from build123d import *

# Parameters (mm, degrees)
SKETCH_W        = 70.3
SKETCH_H        = 51
PAD_DEPTH       = 50.65
SKETCH001_W     = 44.3
SKETCH001_H     = 47.65
SKETCH001_W_2   = 10
POCKET_DEPTH    = 51.001
SKETCH002_R     = 2
SKETCH002_W     = 15
SKETCH002_H     = 15
POCKET001_DEPTH = 50.651


with BuildPart() as part:
    # Sketch → Pad (new body)
    with BuildSketch(Plane.XY):
        with Locations((35.15, 25.5)):
            Rectangle(SKETCH_W, SKETCH_H)
    extrude(amount=PAD_DEPTH)

    # Sketch001 → Pocket (cut, through all)
    with BuildSketch(Plane.XZ):
        with Locations((35.15, 23.825)):
            Rectangle(SKETCH001_W, SKETCH001_H)
        with Locations((5, 26.825)):
            Rectangle(SKETCH001_W_2, SKETCH001_H)
        with Locations((65.3, 26.825)):
            Rectangle(SKETCH001_W_2, SKETCH001_H)
    extrude(amount=-POCKET_DEPTH, mode=Mode.SUBTRACT)

    # Sketch002 → Pocket001 (cut, through all)
    with BuildSketch(Plane.XY.offset(50.65)):
        with Locations((20, 41)):
            Circle(SKETCH002_R)
        with Locations((50.3, 41)):
            Circle(SKETCH002_R)
        with Locations((20, 10)):
            Circle(SKETCH002_R)
        with Locations((50.3, 10)):
            Circle(SKETCH002_R)
        with Locations((4, 40.8)):
            Circle(SKETCH002_R)
        with Locations((4, 30.6)):
            Circle(SKETCH002_R)
        with Locations((4, 20.4)):
            Circle(SKETCH002_R)
        with Locations((4, 10.2)):
            Circle(SKETCH002_R)
        with Locations((66.3, 40.8)):
            Circle(SKETCH002_R)
        with Locations((66.3, 30.6)):
            Circle(SKETCH002_R)
        with Locations((66.3, 20.4)):
            Circle(SKETCH002_R)
        with Locations((66.3, 10.2)):
            Circle(SKETCH002_R)
        with Locations((35.15, 43.5)):
            Rectangle(SKETCH002_W, SKETCH002_H)
    extrude(amount=-POCKET001_DEPTH, mode=Mode.SUBTRACT)


solid = part.part
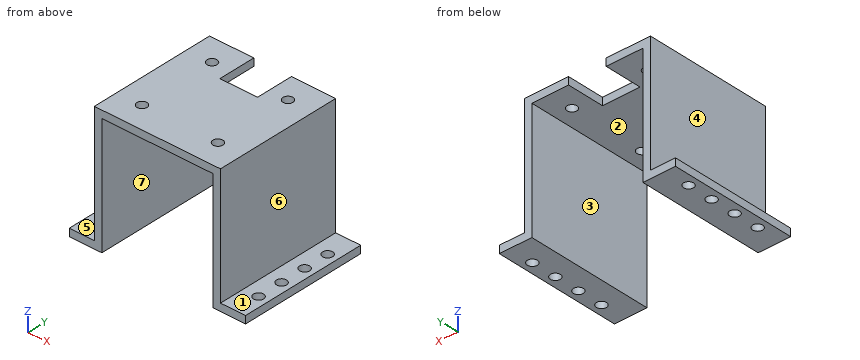
Design review of the part built by this model. Coordinates are the model's own, in mm. Face numbers are marked on the shaded views. A direction names the side the tool comes from. Coordinates: 2 decimals unless noted, no trailing zeros. Order: outer loops, then holes, each group sorted by start corner. A loop starts at its lowest first (then second) coordinate and runs counter-clockwise, first axis right, second up. Notation, with made-up numbers: M 57.25,-16 L 112.25,-16 A26 ccw 112.25,2 Z; hole C -4.75,33 d2. An arc over 180 degrees is marked long. Use a Markdown table: item, result.
(1) Add section C-C (x = 4). Give the boundary of the cut face in (y, z).
Worked answers:
| item | result |
|---|---|
| outline | M 0,0 L 8.2,0 L 8.2,3 L 0,3 Z; M 12.2,0 L 18.4,0 L 18.4,3 L 12.2,3 Z; M 22.4,0 L 28.6,0 L 28.6,3 L 22.4,3 Z; M 32.6,0 L 38.8,0 L 38.8,3 L 32.6,3 Z; M 42.8,0 L 51,0 L 51,3 L 42.8,3 Z |
(2) Draft analysis for pull direction X (two halves, no side actions). For the marked faces 1, 2, 3 and 4, state which applies: released by +X, released by -X, zero draft, split by the parting line, or undercut.
Worked answers:
| item | result |
|---|---|
| face 1 | zero draft |
| face 2 | undercut |
| face 3 | undercut |
| face 4 | released by -X |
(3) Add section B-B (z = 22.5). Give the boundary of the cut face in (x, y), then the cut area to 3 significant figures.
Worked answers:
| item | result |
|---|---|
| outline | M 10,0 L 13,0 L 13,51 L 10,51 Z; M 57.3,0 L 60.3,0 L 60.3,51 L 57.3,51 Z |
| area | 306 mm2 |
(4) Add section D-D (y = 37.5). Give the boundary of the cut face in (x, z).
Worked answers:
| item | result |
|---|---|
| outline | M 0,0 L 13,0 L 13,47.65 L 27.65,47.65 L 27.65,50.65 L 10,50.65 L 10,3 L 0,3 Z; M 42.65,47.65 L 57.3,47.65 L 57.3,0 L 70.3,0 L 70.3,3 L 60.3,3 L 60.3,50.65 L 42.65,50.65 Z |
(5) For the marked faces 5, 6 and 7, list the 3-axis set-ups (+Z, -Z, +X, -X, +Y, -Y) from which the entire face can be reached by the end or side of a thin tool; tool diameter is ignored.
Worked answers:
| item | result |
|---|---|
| face 5 | +Z, -X, +Y, -Y |
| face 6 | +Z, +X, +Y, -Y |
| face 7 | -Z, +Y, -Y |
(6) Add section A-A (y = 30.6). Give the boundary of the cut face in (x, z).
Worked answers:
| item | result |
|---|---|
| outline | M 0,0 L 2,0 L 2,3 L 0,3 Z; M 6,0 L 13,0 L 13,47.65 L 57.3,47.65 L 57.3,0 L 64.3,0 L 64.3,3 L 60.3,3 L 60.3,50.65 L 10,50.65 L 10,3 L 6,3 Z; M 68.3,0 L 70.3,0 L 70.3,3 L 68.3,3 Z |
(7) For P1, Ø10, axis at y = 23.5, z = 16, coming from the -X side; P2, Ø24, axis at y = 17.5, z = 30, coming from the +X side; P3, Ø0.9, axis at x = 34, z = 49, coming from the +Y side; P4, Ø4.5, axis at x = 4, y = 30.6, coming from the -Z side, all flat-tipped, find the tip position at first contact; note any pin that passes through.
Worked answers:
| item | result |
|---|---|
| P1 | stops at x = 10 |
| P2 | stops at x = 60.3 |
| P3 | stops at y = 36 |
| P4 | stops at z = 0 |
(8) Wall thickness on probe 1 along Y at (x, z) = (4, 1.9); probe 2 along X at (y, z) = (15.5, 37); probe 3 along X at (y, z) = (40, 1): over which ranges is each line inside the solid? List them lowest first.
Worked answers:
| item | result |
|---|---|
| probe 1 | y = 0 to 8.2, 12.2 to 18.4, 22.4 to 28.6, 32.6 to 38.8, 42.8 to 51 |
| probe 2 | x = 10 to 13, 57.3 to 60.3 |
| probe 3 | x = 0 to 2.17, 5.83 to 13, 57.3 to 64.47, 68.13 to 70.3 |
